Check sheet for the drawn part. Datum: minimum x, y, z corner. Units: mm. A direction names the side the tool comes from. Round coordinates to 2 decimals unless told otherwise and drop trailing zeros. Write each loop counter-clockwise with the first axis right and the second up, starting at its lowest first coordinate (ties: lowest second). Pieces come first, ordered by that corner, then holes.
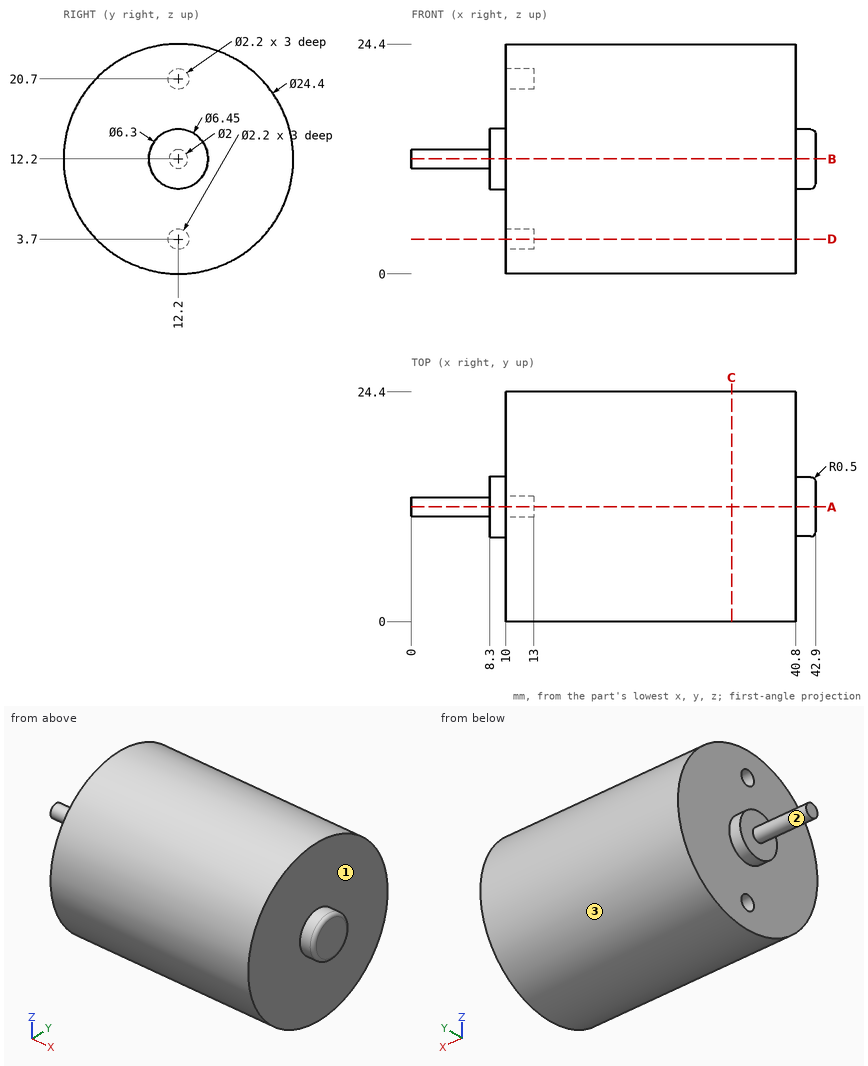
Q1. Material ranges on line 1 along X through (y, z) = (11, 22.75); line 2 along Y through (x, z) = (11.1, 20.7); line 3 along X through (y, z) = (14.25, 11.75), recorded low to high.
Recorded:
line 1: x = 10 to 40.8
line 2: y = 3.45 to 11.1, 13.3 to 20.95
line 3: x = 8.3 to 42.9
Q2. Sectioned sample at C-C (x = 34). Enter the section's corners in (y, z).
Recorded:
outline: circle Ø24.4 at (12.2, 12.2)
Q3. Sectioned sample at D-D (z = 3.7). Enter the section's corners in (x, y).
Recorded:
outline: (10, 3.45) - (40.8, 3.45) - (40.8, 20.95) - (10, 20.95) - (10, 13.3) - (13, 13.3) - (13, 11.1) - (10, 11.1) - close
Q4. Tool access check on the marked faces 1, 2 and 3. Record the directions out of +Z, -Z, +X, -X, +Y, -Y that give a thin tool (end or side, any length) a straight path to the whole face; none if there is none.
Recorded:
face 1: +X
face 2: -X
face 3: +X, -X
Q5. Depth check by flat-ended pin: P1, Ø1.8, axis at y = 12.5, z = 3.5, coming from the -X side; P2, Ø7.5, axis at y = 18, z = 9, coming from the +X side; P3, Ø1, axis at x = 8, y = 15, coming from the -Z side. Enter the tip coordinate at first touch or a pass-through.
Recorded:
P1: stops at x = 10
P2: stops at x = 42.85
P3: stops at z = 10.05
Q6. Sectioned sample at B-B (z = 12.2). Enter the section's corners in (x, y) (3 decimals), plus the area to 3 significant figures.
Recorded:
outline: (0, 11.2) - (8.3, 11.2) - (8.3, 8.975) - (10, 8.975) - (10, 0) - (40.8, 0) - (40.8, 9.05) - (42.4, 9.05) arc R0.5 ccw to (42.9, 9.55) - (42.9, 14.85) arc R0.5 ccw to (42.4, 15.35) - (40.8, 15.35) - (40.8, 24.4) - (10, 24.4) - (10, 15.425) - (8.3, 15.425) - (8.3, 13.2) - (0, 13.2) - close
area: 792 mm2
Q7. Sectioned sample at A-A (y = 12.2). Enter the section's corners in (x, z) (3 decimals), plus the area to 3 significant figures.
Recorded:
outline: (0, 11.2) - (8.3, 11.2) - (8.3, 8.975) - (10, 8.975) - (10, 4.8) - (13, 4.8) - (13, 2.6) - (10, 2.6) - (10, 0) - (40.8, 0) - (40.8, 9.05) - (42.4, 9.05) arc R0.5 ccw to (42.9, 9.55) - (42.9, 14.85) arc R0.5 ccw to (42.4, 15.35) - (40.8, 15.35) - (40.8, 24.4) - (10, 24.4) - (10, 21.8) - (13, 21.8) - (13, 19.6) - (10, 19.6) - (10, 15.425) - (8.3, 15.425) - (8.3, 13.2) - (0, 13.2) - close
area: 779 mm2
